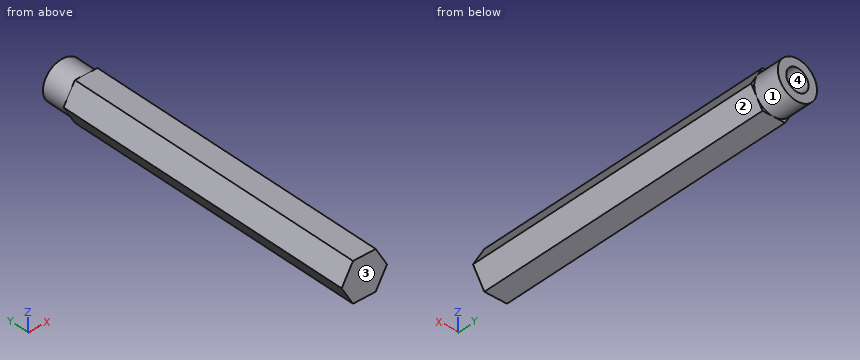
from build123d import *

# Parameters (mm, degrees)
BOSS_EXTRUDE1_DEPTH = 18.6944
SKETCH2_R           = 2.38125
BOSS_EXTRUDE2_DEPTH = 3.175
SKETCH3_R           = 1.35255
CUT_EXTRUDE1_DEPTH  = 6.35


with BuildPart() as part:
    # Sketch1 → Boss-Extrude1 (new body, symmetric)
    with BuildSketch(Plane(origin=(0, 0, 0), x_dir=(1, 0, 0), z_dir=(0, 1, 0))):
        Polygon((1.374815329, -2.38125), (2.749630657, 0), (1.374815329, 2.38125), (-1.374815329, 2.38125), (-2.749630657, 0), (-1.374815329, -2.38125), align=None)
    extrude(amount=BOSS_EXTRUDE1_DEPTH, both=True)

    # Sketch2 → Boss-Extrude2 (add)
    with BuildSketch(Plane(origin=(0, 18.6944, 0), x_dir=(1, 0, 0), z_dir=(0, 1, 0))):
        Circle(SKETCH2_R)
    extrude(amount=BOSS_EXTRUDE2_DEPTH)

    # Sketch3 → Cut-Extrude1 (cut)
    with BuildSketch(Plane(origin=(0, 21.8694, 0), x_dir=(1, 0, 0), z_dir=(0, 1, 0))):
        Circle(SKETCH3_R)
    extrude(amount=-CUT_EXTRUDE1_DEPTH, mode=Mode.SUBTRACT)


solid = part.part
Geometry: final body of the model. Coordinates: model frame, mm. Face numbers are marked on the shaded views. Give positions to 0.01 mm unless a question says otherwise; leave off trailing zeros. Write each loop counter-clockwise with the first axis right and the second up, starting at its lowest first coordinate (ties: lowest second). Pieces come first, ordered by that corner, then holes. Notation, with made-up numbers: (73, 17) -> (87, 17) arc R18 cw to (87, 25) -> close; hole circle Ø6 at (8.5, -8.5). An arc over 180 degrees is marked (long way). Answer as a JSON object with one key per item and string values.
1. Ray query, probe 1 along Z at (x, y) = (0, 17); probe 2 along Y at (x, z) = (-0.3, -0.2). Return the intervals inside material, ascending. Write a range as from..to.
Ans:
{"probe 1": "z = -2.38..-1.35, 1.35..2.38", "probe 2": "y = -18.69..15.52"}
2. Cut plane B-B on y = 3. Output: boundary loops of the cut face in (x, z), and give its area (3 significant figures).
Ans:
{"outline": "(-2.75, 0) -> (-1.37, -2.38) -> (1.37, -2.38) -> (2.75, 0) -> (1.37, 2.38) -> (-1.37, 2.38) -> close", "area": "19.6 mm^2"}
3. Mould query, pull axis Z, two halves, no side actions, for the marked faces 1, 2, 3 and 4. Classes: pulls with the +Z half, pulls with the -Z half, needs draft (parallel to the pull), parting line crosses it, or undercut.
Ans:
{"face 1": "parting line crosses it", "face 2": "pulls with the -Z half", "face 3": "needs draft", "face 4": "undercut"}
4. Contact query for flat-ended pins moving along their axis: pin 1 (0.5 mm diameter, centred on x = 2.5, z = 0, fed in from +Y); pin 2 (1.5 mm diameter, centred on y = 4, z = 0.5, fed in from +X). Output: stop coordinate, or through.
Ans:
{"pin 1": "stops at y = 21.87", "pin 2": "stops at x = 2.75"}
5. Cut plane A-A on z = 0.4. Output: boundary loops of the cut face in (x, y).
Ans:
{"outline": "(-2.52, -18.69) -> (2.52, -18.69) -> (2.52, 18.69) -> (2.35, 18.69) -> (2.35, 21.87) -> (1.29, 21.87) -> (1.29, 15.52) -> (-1.29, 15.52) -> (-1.29, 21.87) -> (-2.35, 21.87) -> (-2.35, 18.69) -> (-2.52, 18.69) -> close"}
